Here's how the part is built. I have some questions about the finished solid (model axes, mm). A direction names the side the tool comes from. Give positions to 0.01 mm unless a question says otherwise; leave off trailing zeros. Write each loop counter-clockwise with the first axis right and the second up, starting at its lowest first coordinate (ties: lowest second). Pieces come first, ordered by that corner, then holes. Notation, with made-up numbers: (32, 51) -> (87, 51) arc R9 ccw to (87, 58) -> close; hole circle Ø1 at (-7, 27.5). An arc over 180 degrees is marked (long way). Put each result on its own line as item: value. Start each with the question number.
from build123d import *

# Parameters (mm, degrees)
BOSS_EXTRUDE1_DEPTH = 5
SKETCH2_R           = 3
SKETCH2_R_2         = 1.5
CUT_EXTRUDE1_DEPTH  = 5
SKETCH3_R           = 6.5
CUT_EXTRUDE2_DEPTH  = 3
CUT_EXTRUDE3_DEPTH  = 3
CUT_EXTRUDE4_DEPTH  = 5


with BuildPart() as part:
    # Sketch1 → Boss-Extrude1 (new body)
    with BuildSketch(Plane.XY):
        with BuildLine():
            Line((40, -15), (55, 0))
            Line((55, 0), (40, 15))
            Line((40, 15), (-50, 15))
            ThreePointArc((-50, 15), (-65, 0), (-50, -15))
            Line((-50, -15), (40, -15))
        make_face()
    extrude(amount=BOSS_EXTRUDE1_DEPTH)

    # Sketch2 → Cut-Extrude1 (cut)
    with BuildSketch(Plane.XY.offset(5)):
        with Locations((-45, 0)):
            Circle(SKETCH2_R)
        with Locations((-28.5, 0)):
            Circle(SKETCH2_R_2)
    extrude(amount=-CUT_EXTRUDE1_DEPTH, mode=Mode.SUBTRACT)

    # Sketch3 → Cut-Extrude2 (cut)
    with BuildSketch(Plane.XY.offset(5)):
        with Locations((-45, 0)):
            Circle(SKETCH3_R)
    extrude(amount=-CUT_EXTRUDE2_DEPTH, mode=Mode.SUBTRACT)

    # Sketch4 → Cut-Extrude3 (cut)
    with BuildSketch(Plane.XY.offset(5)):
        with BuildLine():
            Line((-29.755535663, -4.5), (-60.244464337, -4.5))
            ThreePointArc((-60.244464337, -4.5), (-64.744464337, 0), (-60.244464337, 4.5))
            Line((-60.244464337, 4.5), (-29.755535663, 4.5))
            ThreePointArc((-29.755535663, 4.5), (-25.255535663, 0), (-29.755535663, -4.5))
        make_face()
    extrude(amount=-CUT_EXTRUDE3_DEPTH, mode=Mode.SUBTRACT)

    # Sketch6 → Cut-Extrude4 (cut)
    with BuildSketch(Plane.XY.offset(5)):
        with BuildLine():
            Line((-17.3786019, 4.5), (37.6213981, 4.5))
            ThreePointArc((37.6213981, 4.5), (42.1213981, 0), (37.6213981, -4.5))
            Line((37.6213981, -4.5), (-17.3786019, -4.5))
            ThreePointArc((-17.3786019, -4.5), (-21.8786019, 0), (-17.3786019, 4.5))
        make_face()
    extrude(amount=-CUT_EXTRUDE4_DEPTH, mode=Mode.SUBTRACT)


solid = part.part
1) I'm going to push flat-ended pins straight in: pin 1 Ø7 at (x, y) = (-45, 0) entering from -Z; pin 2 Ø1.5 at (x, z) = (-56.5, 3) entering from +Y; pin 3 Ø0.9 at (x, z) = (-55, 3.5) entering from -Y; pin 4 Ø1 at (y, z) = (-12, 1) entering from -X. Where does each tip first touch, or does it pass through?
2) I want a section at D-D, the plane y = 9.5. Write out the boundary of the cut face in (x, z), and give its area (3 significant figures).
3) I need wall thicknesses on probe 1 along Y at (x, z) = (-45, 1); probe 2 along Y at (x, z) = (25, 2.1); probe 3 along Z at (x, y) = (-48.5, 3). Which ranges of each line are inside material? Lowest first, please.
4) I want a section at C-C, the plane x = -36.5. Write out the boundary of the cut face in (y, z), and give its area (3 significant figures).
5) Which directions (+Z, -Z, +X, -X, +Y, -Y) give clear straight access to the entire face, cutting with the end or side of a thin tool? Please do faces 1 (the flat face through (11, -4.5, 3)), 2 (the flat face through (-35, 4.5, 4)), 3 (the flat face through (47, -8, 2)).
6) I want a section at A-A, the plane z = 3. Write out the boundary of the cut face in (x, y).
7) Thinking about a two-plate mould opening in Y: for faces 4 (the flat face through (-6, 7, 5)), 5 (the cylindrical face through (-44.9, 6.5, 3.5)), 6 (the flat face through (48, 7, 2)), 7 (the cylindrical face through (42.12, 0.1, 2.54)), which applies, released by +Y, released by -Y, zero draft, split by the parting line, or undercut?
8) I want a section at B-B, the plane x = -8.5. Write out the boundary of the cut face in (y, z), and give its area (3 significant figures).
Established:
1. pin 1: stops at z = 0
1. pin 2: stops at y = 13.85
1. pin 3: stops at y = -14.29
1. pin 4: stops at x = -59.63
2. outline: (-61.61, 0) -> (45.5, 0) -> (45.5, 5) -> (-61.61, 5) -> close
2. area: 536 mm2
3. probe 1: y = -15 to -3, 3 to 15
3. probe 2: y = -15 to -4.5, 4.5 to 15
3. probe 3: z = 0 to 2
4. outline: (-15, 0) -> (15, 0) -> (15, 5) -> (4.5, 5) -> (4.5, 2) -> (-4.5, 2) -> (-4.5, 5) -> (-15, 5) -> close
4. area: 123 mm2
5. face 1: +Z, -Z
5. face 2: +Z
5. face 3: +Z, -Z, +X, -Y
6. outline: (-50, -15) -> (40, -15) -> (55, 0) -> (40, 15) -> (-50, 15) arc R15 ccw to start; hole (-60.24, -4.5) -> (-49.69, -4.5) arc R6.5 ccw to (-40.31, -4.5) -> (-29.76, -4.5) arc R4.5 ccw to (-29.76, 4.5) -> (-40.31, 4.5) arc R6.5 ccw to (-49.69, 4.5) -> (-60.24, 4.5) arc R4.5 ccw to start; hole (-17.38, -4.5) -> (37.62, -4.5) arc R4.5 ccw to (37.62, 4.5) -> (-17.38, 4.5) arc R4.5 ccw to start
7. face 4: zero draft
7. face 5: undercut
7. face 6: released by +Y
7. face 7: undercut
8. outline: (-15, 0) -> (-4.5, 0) -> (-4.5, 5) -> (-15, 5) -> close; (4.5, 0) -> (15, 0) -> (15, 5) -> (4.5, 5) -> close
8. area: 105 mm2
